```python
from build123d import *

# Parameters (mm, degrees)
SKETCH1_W                   = 15.24
SKETCH1_H                   = 25.4
BOSS_EXTRUDE1_DEPTH         = 6.35
F_29_0_136_DIAMETER_HOLE1_D = 3.4544
SKETCH6_R                   = 1.45
CUT_EXTRUDE1_DEPTH          = 16.24


with BuildPart() as part:
    # Sketch1 → Boss-Extrude1 (new body)
    with BuildSketch(Plane.XY):
        Rectangle(SKETCH1_W, SKETCH1_H)
    extrude(amount=BOSS_EXTRUDE1_DEPTH)

    # #29 (0.136) Diameter Hole1 (through all)
    with Locations(Plane.XY.offset(6.35)):
        with Locations((0, -7.62), (0, 7.62)):
            Hole(F_29_0_136_DIAMETER_HOLE1_D / 2)

    # Sketch6 → Cut-Extrude1 (cut, through all)
    with BuildSketch(Plane.ZY.offset(7.62)):
        Circle(SKETCH6_R)
    extrude(amount=-CUT_EXTRUDE1_DEPTH, mode=Mode.SUBTRACT)


solid = part.part
```
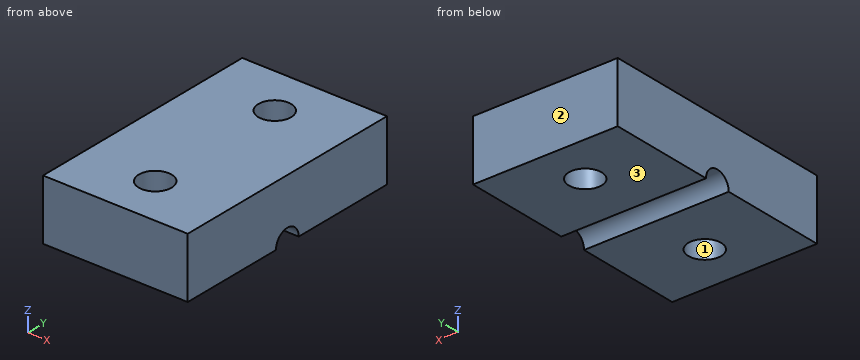
CAD build for the part. Positions are in the model's coordinates, mm. Face numbers are marked on the shaded views. Round coordinates to 2 decimals unless told otherwise and drop trailing zeros. Order: outer loops, then holes, each group sorted by start corner. A loop starts at its lowest first (then second) coordinate and runs counter-clockwise, first axis right, second up.
Q1. Two-plate mould, pull along Y, no slides. Class the marked faces 1, 2 and 3: pulls with the +Y half, pulls with the -Y half, needs draft (parallel to the pull), parting line crosses it, or undercut.
Q2. Slice it at D-D (x = 4). Write the cut outline in (y, z), and give its area (3 significant figures).
Q3. Wall check: L1, parallel to Y at x = 0, z = 3.25; L2, parallel to Y at x = 0.75, z = 5.5; L3, parallel to X at y = 6.25, z = 5.75. Give the ranges that are in metal, low to high.
Q4. Slice it at B-B (x = 0). Write the cut outline in (y, z).
Q5. Drop a flat-ended pin along its axis: pin 1 (4.5 mm diameter, centred on x = 0, y = -7.62, fed in from -Z). Give the stop position or say it passes through.
Q6. Slice it at C-C (z = 3.25). Write the cut outline in (x, y).
Q7. Slice it at A-A (y = -7.62). Write the cut outline in (x, z).
Results below:
1. face 1: undercut
1. face 2: pulls with the +Y half
1. face 3: needs draft
2. outline: (-12.7, 0) - (-1.45, 0) arc R1.45 cw to (1.45, 0) - (12.7, 0) - (12.7, 6.35) - (-12.7, 6.35) - close
2. area: 158 mm2
3. L1: y = -12.7 to -9.35, -5.89 to 5.89, 9.35 to 12.7
3. L2: y = -12.7 to -9.18, -6.06 to 6.06, 9.18 to 12.7
3. L3: x = -7.62 to -1.05, 1.05 to 7.62
4. outline: (-12.7, 0) - (-9.35, 0) - (-9.35, 6.35) - (-12.7, 6.35) - close; (-5.89, 0) - (-1.45, 0) arc R1.45 cw to (1.45, 0) - (5.89, 0) - (5.89, 6.35) - (-5.89, 6.35) - close; (9.35, 0) - (12.7, 0) - (12.7, 6.35) - (9.35, 6.35) - close
5. pin 1: stops at z = 0
6. outline: (-7.62, -12.7) - (7.62, -12.7) - (7.62, 12.7) - (-7.62, 12.7) - close; hole circle Ø3.45 at (0, -7.62); hole circle Ø3.45 at (0, 7.62)
7. outline: (-7.62, 0) - (-1.73, 0) - (-1.73, 6.35) - (-7.62, 6.35) - close; (1.73, 0) - (7.62, 0) - (7.62, 6.35) - (1.73, 6.35) - close
